The figure shows three views and two pictorial views of one solid part (mm, origin at its lowest corner). Answer the questions. A direction names the side the tool comes from. Coordinates: 2 decimals unless noted, no trailing zeros. Order: outer loops, then holes, each group sorted by start corner. A loop starts at its lowest first (then second) coordinate and runs counter-clockwise, first axis right, second up.
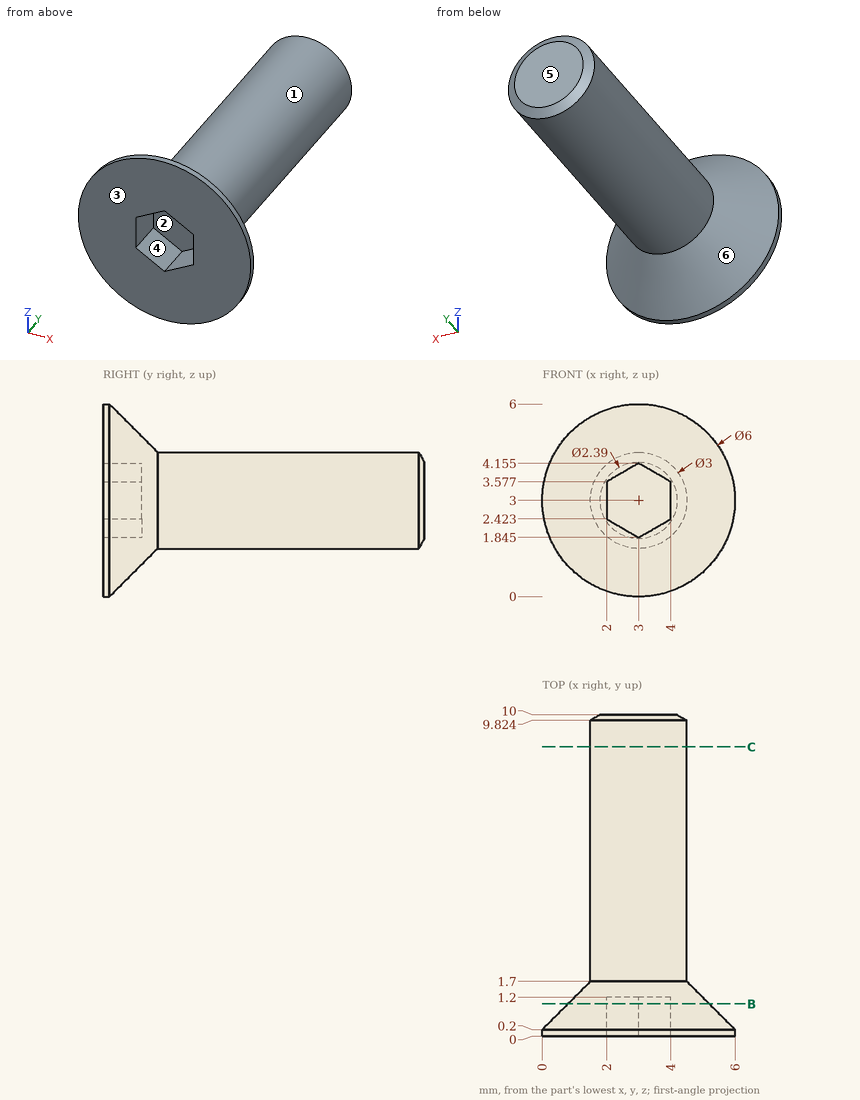
Q1. The part is cut by section B-B, the plane y = 1. Determine the outline of the cut face in (x, z) (1 decimal).
Q2. Determine the mould class of the marked faces 4, 5 and 6 for opening direction Z: +Z half, -Z half, draft (parallel to the pull), parting line (faces both ways), or undercut.
Q3. Which of the six approach directions +Z, -Z, +X, -X, +Y, -Y give full straight-line access (tool end or side, diameter ignored) to the marked faces 1, 2 and 3?
Q4. Straight lines are drawn through the part: L1, parallel to X at y = 1, z = 3.7 (1 decimal); L2, parallel to Y at x = 2.8, z = 3.3; L3, parallel to Y at x = 0.8, z = 1.1. For each, find the intervals that lie inside material, in ascending order.
Q5. The part is cut by section C-C, the plane y = 9. Determine the outline of the cut face in (x, z).
Q6. Each of these flat-tipped pins is pushed along its axis until it touches: P1, Ø1.5, axis at x = 4.5, y = 5.5, coming from the -Z side; P2, Ø3, axis at x = 2, y = 7.5, coming from the +Z side. Where does it stop, or does it pass through?
Computed values:
1. outline: circle Ø4.4 at (3, 3); hole (2, 2.4) - (3, 1.8) - (4, 2.4) - (4, 3.6) - (3, 4.2) - (2, 3.6) - close
2. face 4: undercut
2. face 5: draft
2. face 6: parting line
3. face 1: +Y
3. face 2: -Y
3. face 3: +Z, -Z, +X, -X, -Y
4. L1: x = 0.9 to 2.2, 3.8 to 5.1
4. L2: y = 1.2 to 10
4. L3: y = 0 to 0.29
5. outline: circle Ø3 at (3, 3)
6. P1: stops at z = 1.7
6. P2: stops at z = 4.5
